from build123d import *

# Parameters (mm, degrees)
BOSS_EXTRUDE1_DEPTH = 4
SKETCH2_R           = 1.75
CUT_EXTRUDE1_DEPTH  = 202.161626559
SKETCH3_R           = 1.75
CUT_EXTRUDE2_DEPTH  = 202.161626559
SKETCH4_R           = 1.75
CUT_EXTRUDE3_DEPTH  = 202.161626559
SKETCH5_R           = 1.75
CUT_EXTRUDE4_DEPTH  = 202.161626559


with BuildPart() as part:
    # Sketch1 → Boss-Extrude1 (new body)
    with BuildSketch(Plane(origin=(0, 0, 0), x_dir=(1, 0, 0), z_dir=(0, 1, 0))):
        Polygon((-90, 30), (-15, 105), (-15, 138), (-115, 150), (-115, 165), (115, 165), (115, 150), (15, 138), (15, 105), (90, 30), (90, -30), (-90, -30), align=None)
    extrude(amount=BOSS_EXTRUDE1_DEPTH)

    # Sketch2 → Cut-Extrude1 (cut, through all)
    with BuildSketch(Plane(origin=(0, 4, 0), x_dir=(1, 0, 0), z_dir=(0, 1, 0))):
        with Locations(Location((-85, 25, 0), (0, 0, 270))):
            Circle(SKETCH2_R)
        with Locations(Location((85, 25, 0), (0, 0, 90))):
            Circle(SKETCH2_R)
        with Locations(Location((85, -25, 0), (0, 0, 270))):
            Circle(SKETCH2_R)
        with Locations(Location((-85, -25, 0), (0, 0, 90))):
            Circle(SKETCH2_R)
        with Locations(Location((-70, 25, 0), (0, 0, 270))):
            Circle(SKETCH2_R)
        with Locations(Location((-70, -25, 0), (0, 0, 90))):
            Circle(SKETCH2_R)
        with Locations(Location((70, -25, 0), (0, 0, 270))):
            Circle(SKETCH2_R)
        with Locations(Location((70, 25, 0), (0, 0, 90))):
            Circle(SKETCH2_R)
    extrude(amount=-CUT_EXTRUDE1_DEPTH, mode=Mode.SUBTRACT)

    # Sketch3 → Cut-Extrude2 (cut, through all)
    with BuildSketch(Plane(origin=(0, 4, 0), x_dir=(1, 0, 0), z_dir=(0, 1, 0))):
        with Locations(Location((2.4, 76.6, 0), (0, 0, 270))):
            Circle(SKETCH3_R)
        with Locations(Location((-33.8, 42.3, 0), (0, 0, 270))):
            Circle(SKETCH3_R)
        with Locations(Location((33.9, 76.6, 0), (0, 0, 270))):
            Circle(SKETCH3_R)
        with Locations(Location((29.5, 42.3, 0), (0, 0, 270))):
            Circle(SKETCH3_R)
    extrude(amount=-CUT_EXTRUDE2_DEPTH, mode=Mode.SUBTRACT)

    # Sketch4 → Cut-Extrude3 (cut, through all)
    with BuildSketch(Plane(origin=(0, 4, 0), x_dir=(1, 0, 0), z_dir=(0, 1, 0))):
        with Locations(Location((-23.9, -0.6, 0), (0, 0, 270))):
            Circle(SKETCH4_R)
        with Locations(Location((-8.9, -0.6, 0), (0, 0, 270))):
            Circle(SKETCH4_R)
        with Locations(Location((8.9, -0.6, 0), (0, 0, 270))):
            Circle(SKETCH4_R)
        with Locations(Location((23.9, -0.6, 0), (0, 0, 270))):
            Circle(SKETCH4_R)
    extrude(amount=-CUT_EXTRUDE3_DEPTH, mode=Mode.SUBTRACT)

    # Sketch5 → Cut-Extrude4 (cut, through all)
    with BuildSketch(Plane(origin=(0, 4, 0), x_dir=(1, 0, 0), z_dir=(0, 1, 0))):
        with Locations(Location((0, 157, 0), (0, 0, 270))):
            Circle(SKETCH5_R)
        with Locations(Location((-30, 157, 0), (0, 0, 270))):
            Circle(SKETCH5_R)
        with Locations(Location((30, 157, 0), (0, 0, 270))):
            Circle(SKETCH5_R)
        with Locations(Location((80, 157, 0), (0, 0, 270))):
            Circle(SKETCH5_R)
        with Locations(Location((-80, 157, 0), (0, 0, 270))):
            Circle(SKETCH5_R)
    extrude(amount=-CUT_EXTRUDE4_DEPTH, mode=Mode.SUBTRACT)


solid = part.part
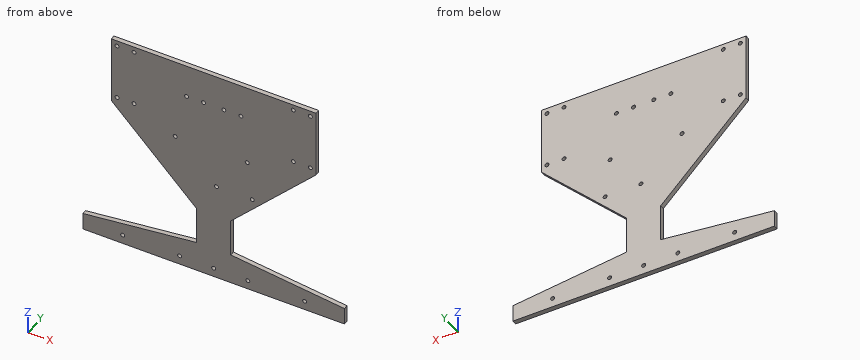
Verification items for the finished model (mm, model axes). Coordinates: 2 decimals unless noted, no trailing zeros. Order: outer loops, then holes, each group sorted by start corner. A loop starts at its lowest first (then second) coordinate and runs counter-clockwise, first axis right, second up. Notation, with made-up numbers: M 9,33 L 66,33 A11 cw 66,53 Z; hole C 65,-17.5 d9. An arc over 180 degrees is marked long. One line per item, written item: value. Start each with the question number.
Item 1: Scan lines: probe 1 along X at (y, z) = (1.2, -157); probe 2 along X at (y, z) = (2.45, 0.6); probe 3 along Z at (x, y) = (85, 2.15). Record each from-to range of solid material in increasing order.
Item 2: Sectioned sample at A-A (y = 3.2). Count the separate pieces of the cut face and the enclosed holes in it, then the cut area to 3 significant figures.
Item 3: Sectioned sample at B-B (x = -75.5). Enter the section's corners in (y, z).
Item 4: Sectioned sample at C-C (z = -12). Enter the section's corners in (x, y), then the cut area to 3 significant figures.
Item 5: Sectioned sample at D-D (z = -57.5). Enter the section's corners in (x, y).
Item 6: Gauge pin test, flat ends, axial feed: pin 1 (2 mm diameter, centred on y = 1.5, z = 15, fed in from +X); pin 2 (1.2 mm diameter, centred on y = 2.5, z = -122.5, fed in from +X). Record the tip position at first contact, or that the pin passes through.
Conclusion:
1. probe 1: x = -115 to -81.75, -78.25 to -31.75, -28.25 to -1.75, 1.75 to 28.25, 31.75 to 78.25, 81.75 to 115
1. probe 2: x = -90 to -25.65, -22.15 to -10.65, -7.15 to 7.15, 10.65 to 22.15, 25.65 to 90
1. probe 3: z = -165 to -146.4, -35 to -26.75, -23.25 to 23.25, 26.75 to 30
2. separate pieces: 1
2. enclosed holes: 21
2. area: 24,500 mm^2
3. outline: M 0,-165 L 4,-165 L 4,-145.26 L 0,-145.26 Z; M 0,-44.5 L 4,-44.5 L 4,30 L 0,30 Z
4. outline: M -90,0 L 90,0 L 90,4 L -90,4 Z
4. area: 720 mm^2
5. outline: M -62.5,0 L 62.5,0 L 62.5,4 L -62.5,4 Z
6. pin 1: stops at x = 90
6. pin 2: stops at x = 15
